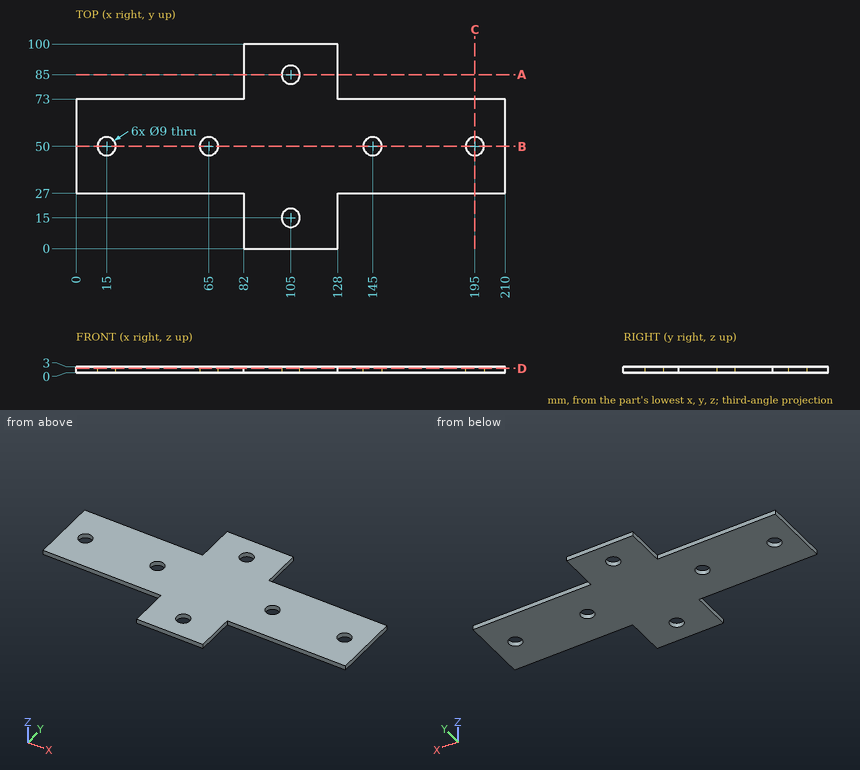
Source: three-view drawing plus pictorial views. Frame: mm from the lowest corner of the part. Round coordinates to 2 decimals unless told otherwise and drop trailing zeros. Loops run counter-clockwise (first coordinate to the right, second up) from the corner with the lowest first, then second, coordinate; pieces in that order, holes last.
Q1. Section B-B, the plane y = 50. Return loops of the section in (x, z).
Q2. Section A-A, the plane y = 85. Return loops of the section in (x, z), plus the area to 3 significant figures.
Q3. Ray query, line 1 (Y direction, x = 105, z = 0.75); line 2 (Y direction, x = 65, z = 1.9); line 3 (Y direction, x = 101, z = 1.2). Return the intervals inside material, ascending.
Q4. Section C-C, the plane x = 195. Return loops of the section in (y, z), plus the area to 3 significant figures.
Q5. Section D-D, the plane z = 2.05. Return loops of the section in (x, y).
Q6. First-contact query: P1, Ø5.5, axis at x = 195, y = 50, coming from the -Z side; P2, Ø1, axis at y = 85.5, z = 2, coming from the +X side; P3, Ø1.5, axis at x = 27.5, z = 1.5, coming from the -Y side. Flat tips, straight axial feed; report the tip coordinate or a pass-through.
Solutions:
1. outline: (0, 0) - (10.5, 0) - (10.5, 3) - (0, 3) - close; (19.5, 0) - (60.5, 0) - (60.5, 3) - (19.5, 3) - close; (69.5, 0) - (140.5, 0) - (140.5, 3) - (69.5, 3) - close; (149.5, 0) - (190.5, 0) - (190.5, 3) - (149.5, 3) - close; (199.5, 0) - (210, 0) - (210, 3) - (199.5, 3) - close
2. outline: (82, 0) - (100.5, 0) - (100.5, 3) - (82, 3) - close; (109.5, 0) - (128, 0) - (128, 3) - (109.5, 3) - close
2. area: 111 mm2
3. line 1: y = 0 to 10.5, 19.5 to 80.5, 89.5 to 100
3. line 2: y = 27 to 45.5, 54.5 to 73
3. line 3: y = 0 to 12.94, 17.06 to 82.94, 87.06 to 100
4. outline: (27, 0) - (45.5, 0) - (45.5, 3) - (27, 3) - close; (54.5, 0) - (73, 0) - (73, 3) - (54.5, 3) - close
4. area: 111 mm2
5. outline: (0, 27) - (82, 27) - (82, 0) - (128, 0) - (128, 27) - (210, 27) - (210, 73) - (128, 73) - (128, 100) - (82, 100) - (82, 73) - (0, 73) - close; hole circle Ø9 at (15, 50); hole circle Ø9 at (65, 50); hole circle Ø9 at (105, 15); hole circle Ø9 at (105, 85); hole circle Ø9 at (145, 50); hole circle Ø9 at (195, 50)
6. P1: passes through
6. P2: stops at x = 128
6. P3: stops at y = 27
